Autodesk Inventor part; units mm, degrees
ref_plane "YZ Plane" through (0, 0, 0) normal (1, 0, 0) x (0, 1, 0)
ref_plane "XZ Plane" through (0, 0, 0) normal (0, 1, 0) x (-1, 0, 0)
ref_plane "XY Plane" through (0, 0, 0) normal (0, 0, 1) x (1, 0, 0)
sketch "Sketch1" plane through (0, 0, 0) normal (0, 0, 1) x (1, 0, 0)
  line L0 (5.7625, -10.525) -> (-5.7625, -10.525)
  line L1 (-5.7625, -10.525) -> (-5.7625, 10.525)
  line L2 (-5.7625, 10.525) -> (5.7625, 10.525)
  line L3 (5.7625, 10.525) -> (5.7625, -10.525)
  point P0 (0, 0)
  dimension "d2" = 21.05
  dimension "d4" = 10.525
  dimension "d7" = 11.525
  dimension "d8" = 5.7625
extrude "Extrusion1" add sketch "Sketch1" against normal blind 127
sketch "Sketch2" plane through (0, 0, 0) normal (0, 0, 1) x (1, 0, 0)
  line L0 (5.7625, -10.525) -> (-5.7625, -10.525)
  line L1 (5.7625, 10.525) -> (5.7625, -10.525)
  line L2 (-5.7625, 10.525) -> (5.7625, 10.525)
  line L3 (-5.7625, -10.525) -> (-5.7625, 10.525)
  line L4 (-4.7625, 9.525) -> (4.7625, 9.525)
  line L5 (4.7625, 9.525) -> (4.7625, -9.525)
  line L6 (4.7625, -9.525) -> (-4.7625, -9.525)
  line L7 (-4.7625, -9.525) -> (-4.7625, 9.525)
  point P0 (0, 0)
  dimension "d11" = 1
  dimension "d12" = 1
  dimension "d13" = 1
  dimension "d14" = 1
extrude "Extrusion2" cut sketch "Sketch2" against normal blind 125 contours L4 L5 L6 L7
equation "\"d2\" = 2 * d4"
equation "\"d12\" = d11"
equation "\"d13\" = d11"
equation "\"d14\" = d11"
properties part number "Waveguide Terminator"
Can you work these out from the model? Positions are in its coordinate system, mm. A direction names the side the tool comes from. Round coordinates to 2 decimals unless told otherwise and drop trailing zeros. Loops run counter-clockwise (first coordinate to the right, second up) from the corner with the lowest first, then second, coordinate; pieces in that order, holes last.
Item 1: Suppose I cut it at A-A, the plane z = -66.5. Write out the boundary of the cut face in (x, y) (1 decimal), then the cut area to 4 significant figures.
Item 2: Which directions (+Z, -Z, +X, -X, +Y, -Y) give clear straight access to the entire face, cutting with the end or side of a thin tool? Please do faces 1 (the flat face through (-5.762, 0, -63)), 2 (the flat face through (0, -9.525, -62)).
Item 3: Suppose I cut it at B-B, the plane y = -2.5. Write out the boundary of the cut face in (x, z).
Item 4: If we mould it in two halves opening along X, with no side actions, what happens to faces 3 (the flat face through (-5, 1, 0)), 4 (the flat face through (-4.762, 0, -62)), 5 (the flat face through (5.762, 0, -63))? For each: +X half, -X half, draft (parallel to the pull), parting line (faces both ways), or undercut.
Item 5: Please list where these lines run through material, in increasing order: L1, parallel to Y at x = -2.25, z = -58.5 (3 decimals); L2, parallel to X at y = -4.5, z = -120.5; L3, parallel to Z at x = -2.25, y = 6.5.
Item 6: Suppose I cut it at C-C, the plane x = -0.5. Write out the boundary of the cut face in (y, z) (3 decimals), then the cut area to 3 significant figures.
Reported:
1. outline: (-5.8, -10.5) - (5.8, -10.5) - (5.8, 10.5) - (-5.8, 10.5) - close; hole (-4.8, -9.5) - (4.8, -9.5) - (4.8, 9.5) - (-4.8, 9.5) - close
1. area: 61.15 mm2
2. face 1: +Z, -Z, -X, +Y, -Y
2. face 2: +Z
3. outline: (-5.76, -127) - (5.76, -127) - (5.76, 0) - (4.76, 0) - (4.76, -125) - (-4.76, -125) - (-4.76, 0) - (-5.76, 0) - close
4. face 3: draft
4. face 4: undercut
4. face 5: +X half
5. L1: y = -10.525 to -9.525, 9.525 to 10.525
5. L2: x = -5.76 to -4.76, 4.76 to 5.76
5. L3: z = -127 to -125
6. outline: (-10.525, -127) - (10.525, -127) - (10.525, 0) - (9.525, 0) - (9.525, -125) - (-9.525, -125) - (-9.525, 0) - (-10.525, 0) - close
6. area: 292 mm2
